Geometry: final body of the model. Coordinates: model frame, mm. Give positions to 0.01 mm unless a question says otherwise; leave off trailing zeros. Write each loop counter-clockwise with the first axis right and the second up, starting at its lowest first coordinate (ties: lowest second). Pieces come first, ordered by that corner, then holes.
```python
from build123d import *

# Parameters (mm, degrees)
F0_W     = 5
F0_H     = 100
F1_DEPTH = 75
F3_DEPTH = 5
F4_DEPTH = 5


with BuildPart() as f1:
    # F0 (on Front) → F1 (new body)
    with BuildSketch(Plane.XZ):
        with Locations((2.5, 50)):
            Rectangle(F0_W, F0_H)
    extrude(amount=F1_DEPTH)

    # F2 (on face) → F3 (cut)
    with BuildSketch(Plane(origin=(0, 0, 0), x_dir=(0, -1, 0), z_dir=(-1, 0, 0))):
        Polygon((75, 100), (15, 100), (75, 20), align=None)
    extrude(amount=-F3_DEPTH, mode=Mode.SUBTRACT)

    # F4 (cut): a face of the model
    f4_faces = [f1.faces().sort_by_distance(p)[0] for p in [
        (2.5, 0, 50),
    ]]
    extrude(f4_faces, amount=-F4_DEPTH, mode=Mode.SUBTRACT)


solid = f1.part
```
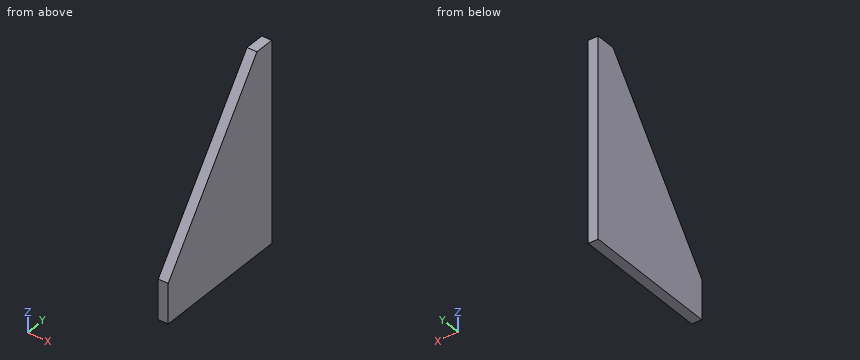
Item 1: Section C-C, the plane y = -36. Return the cut outline in (x, z), plus the area to 3 significant figures.
Found:
outline: (0, 0) - (5, 0) - (5, 72) - (0, 72) - close
area: 360 mm2
Item 2: Section A-A, the plane x = 1.8. Return the cut outline in (y, z).
Found:
outline: (-75, 0) - (-5, 0) - (-5, 100) - (-15, 100) - (-75, 20) - close
Item 3: Section B-B, the plane z = 70. Return the cut outline in (x, y).
Found:
outline: (0, -37.5) - (5, -37.5) - (5, -5) - (0, -5) - close
Item 4: Line query: L1, parallel to Y at x = 2.7, z = 64; L2, parallel to Z at x = 1.9, y = -55.5; L3, parallel to Z at x = 2.2, y = -53.5. Output: solid intervals per line, ascending.
Found:
L1: y = -42 to -5
L2: z = 0 to 46
L3: z = 0 to 48.67
Item 5: Pin query (flat end, axial travel): pin 1 Ø3 at (x, y) = (1, -23.5) entering from +Z; pin 2 Ø2 at (x, y) = (1.5, -43.5) entering from +Z. Return the tip coordinate at first contact, or that it passes through.
Found:
pin 1: stops at z = 90.67
pin 2: stops at z = 63.33
